Geometry: final body of the model. Coordinates: model frame, mm. Round coordinates to 2 decimals unless told otherwise and drop trailing zeros. Loops run counter-clockwise (first coordinate to the right, second up) from the corner with the lowest first, then second, coordinate; pieces in that order, holes last. Notation, with made-up numbers: M -15,36.25 L 39,36.25 A15 ccw 39,52.25 Z; hole C 7.5,84.5 d8. An arc over 180 degrees is marked long. Answer as a JSON object with one key per item and string values.
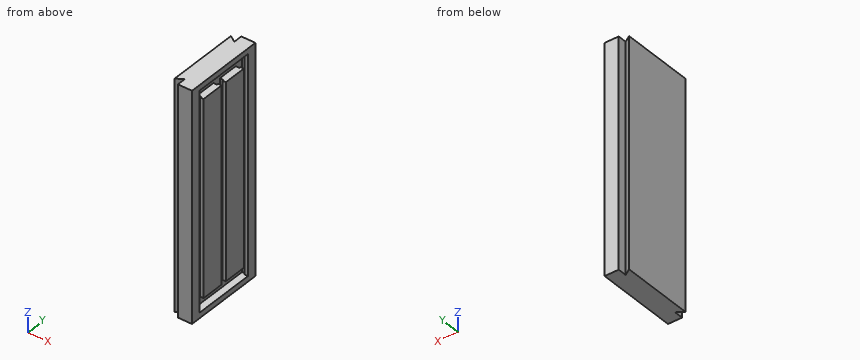
```python
from build123d import *

# Parameters (mm, degrees)
BOSS_EXTRUDE1_DEPTH = 250
CUT_EXTRUDE1_DEPTH  = 238
SKETCH3_W           = 24.5
SKETCH3_H           = 138
CUT_EXTRUDE2_DEPTH  = 15.5


with BuildPart() as part:
    # Sketch1 → Boss-Extrude1 (new body, symmetric)
    with BuildSketch(Plane.XY):
        Polygon((-46, 80), (-46, -80), (-31, -70), (-31, -90), (0, -90), (0, 90), (-31, 90), (-31, 70), align=None)
    extrude(amount=BOSS_EXTRUDE1_DEPTH, both=True)

    # Sketch2 → Cut-Extrude1 (cut, symmetric)
    with BuildSketch(Plane.XY):
        Polygon((0, 69), (-7.5, 69), (-7.5, 72), (-15.5, 72), (-15.5, 54), (-7.5, 54), (-7.5, 57), (0, 57), align=None)
        Polygon((0, 6), (-7.5, 6), (-7.5, 9), (-15.5, 9), (-15.5, -9), (-7.5, -9), (-7.5, -6), (0, -6), align=None)
        Polygon((0, -69), (-7.5, -69), (-7.5, -72), (-15.5, -72), (-15.5, -54), (-7.5, -54), (-7.5, -57), (0, -57), align=None)
    extrude(amount=CUT_EXTRUDE1_DEPTH, both=True, mode=Mode.SUBTRACT)

    # Sketch3 → Cut-Extrude2 (cut)
    with BuildSketch(Plane(origin=(0, 0, 0), x_dir=(0, 0, -1), z_dir=(1, 0, 0))):
        with Locations((-225.75, 0)):
            Rectangle(SKETCH3_W, SKETCH3_H)
        with Locations((225.75, 0)):
            Rectangle(SKETCH3_W, SKETCH3_H)
    extrude(amount=-CUT_EXTRUDE2_DEPTH, mode=Mode.SUBTRACT)


solid = part.part
```
1) Cut plane C-C on x = -36. Return the cut outline in (y, z).
Geometry results:
{"outline": "M -73.33,-250 L 73.33,-250 L 73.33,250 L -73.33,250 Z"}
2) First-contact query: pin 1 (1.5 mm diameter, centred on x = -39, z = 182.5, fed in from -Y). Flat tip, straight axial feed; report the tip coordinate or a pass-through.
Geometry results:
{"pin 1": "y = -75.83"}
3) Cut plane B-B on y = 41. Return the cut outline in (x, z).
Geometry results:
{"outline": "M -46,-250 L 0,-250 L 0,-238 L -15.5,-238 L -15.5,-213.5 L 0,-213.5 L 0,213.5 L -15.5,213.5 L -15.5,238 L 0,238 L 0,250 L -46,250 Z"}
4) Line query: probe 1 along Y at (x, z) = (-4.5, -111); probe 2 along Z at (x, y) = (-13, 47.5); probe 3 along Y at (x, z) = (-11.5, -130.5). Output: solid intervals per line, ascending.
Geometry results:
{"probe 1": "-90 to -69, -57 to -6, 6 to 57, 69 to 90", "probe 2": "-250 to -238, -213.5 to 213.5, 238 to 250", "probe 3": "-90 to -72, -54 to -9, 9 to 54, 72 to 90"}
